Geometry: final body of the model. Coordinates: model frame, mm. Coordinates: 2 decimals unless noted, no trailing zeros. Write each loop counter-clockwise with the first axis right and the second up, starting at its lowest first coordinate (ties: lowest second). Pieces come first, ordered by that corner, then holes. Notation, with made-up numbers: (60, -15.5) - (87, -15.5) arc R30 cw to (87, 7.5) - close; hole circle Ø6 at (62, 1). An arc over 180 degrees is marked (long way). Answer as a JSON object with one key per item and string values. Group by question number.
Item 1: Section C-C on z = 40. State how many separate pieces and enclosed holes the cut face has, and give its area (3 significant figures).
Item 2: Section B-B on x = -12.75. Return loops of the section in (y, z).
Item 3: Line query: line 1 along Y through (x, z) = (-44, 44); line 2 along X through (y, z) = (-11, 47.5); line 3 along X through (y, z) = (-14.5, 12). Output: solid intervals per line, ascending. Write a range as from..to.
Item 4: Mould query, pull axis X, two halves, no side actions, for faces 1 (the cylindrical face through (-55.859, 19.961, 1.203)), 2 (the cylindrical face through (-1.203, -20.859, 36.448)), 3 (the cylindrical face through (-10.766, -14.521, 33.524)). Classes: pulls with the +X half, pulls with the -X half, needs draft (parallel to the pull), parting line crosses it, or undercut.
Item 5: Section A-A on y = 32. Return loops of the section in (x, z).
```python
from build123d import *

# Parameters (mm, degrees)
F0_R     = 2.5
F1_DEPTH = 68
F2_R     = 4


with BuildPart() as f1:
    # F0 (on Top) → F1 (new body)
    with BuildSketch(Plane.XY):
        with BuildLine():
            Line((-44.25, -10.5), (-44.25, 0))
            Line((-44.25, 0), (-57, 0))
            Line((-57, 0), (-57, -22))
            Line((-57, -22), (0, -22))
            Line((0, -22), (0, 0))
            Line((0, 0), (-28.5, 0))
            Line((-28.5, 0), (-28.5, -13))
            Line((-28.5, -13), (-41.75, -13))
            ThreePointArc((-41.75, -13), (-46.017766953, -14.767766953), (-44.25, -10.5))
        make_face()
        with BuildLine():
            ThreePointArc((-10.25, -13), (-12.75, -15.5), (-15.25, -13))
            ThreePointArc((-15.25, -13), (-12.75, -10.5), (-10.25, -13))
        make_face(mode=Mode.SUBTRACT)
        with BuildLine():
            Line((-44.25, 6.5), (-44.25, 0))
            Line((-44.25, 0), (-28.5, 0))
            Line((-28.5, 0), (0, 0))
            Line((0, 0), (0, 63))
            Line((0, 63), (-57, 63))
            Line((-57, 63), (-57, 9))
            Line((-57, 9), (-46.75, 9))
            ThreePointArc((-46.75, 9), (-44.25, 11.5), (-41.75, 9))
            ThreePointArc((-41.75, 9), (-42.482233047, 7.232233047), (-44.25, 6.5))
        make_face()
        with Locations((-12.75, 9.2245186158)):
            Circle(F0_R, mode=Mode.SUBTRACT)
        with Locations((-44.25, 32)):
            Circle(F0_R, mode=Mode.SUBTRACT)
        with BuildLine():
            ThreePointArc((-46.75, 54.2245186158), (-44.25, 56.7245186158), (-41.75, 54.2245186158))
            ThreePointArc((-41.75, 54.2245186158), (-44.25, 51.7245186158), (-46.75, 54.2245186158))
        make_face(mode=Mode.SUBTRACT)
        with Locations((-12.75, 32)):
            Circle(F0_R, mode=Mode.SUBTRACT)
        with BuildLine():
            ThreePointArc((-15.25, 54.2245186158), (-12.75, 56.7245186158), (-10.25, 54.2245186158))
            ThreePointArc((-10.25, 54.2245186158), (-12.75, 51.7245186158), (-15.25, 54.2245186158))
        make_face(mode=Mode.SUBTRACT)
        with BuildLine():
            Line((-57, 0), (-44.25, 0))
            Line((-44.25, 0), (-44.25, 6.5))
            ThreePointArc((-44.25, 6.5), (-46.017766953, 7.232233047), (-46.75, 9))
            Line((-46.75, 9), (-57, 9))
            Line((-57, 9), (-57, 0))
        make_face()
        with BuildLine():
            Line((-28.5, 0), (-44.25, 0))
            Line((-44.25, 0), (-44.25, -10.5))
            ThreePointArc((-44.25, -10.5), (-42.482233047, -11.232233047), (-41.75, -13))
            Line((-41.75, -13), (-28.5, -13))
            Line((-28.5, -13), (-28.5, 0))
        make_face()
    extrude(amount=F1_DEPTH)

    # F2
    f2_edges = [f1.edges().sort_by_distance(p)[0] for p in [
        (-28.5, 63, 0),
        (0, 20.5, 0),
        (-57, 20.5, 0),
        (-57, 63, 34),
        (0, 63, 34),
        (-28.5, -22, 0),
        (-57, -22, 34),
        (0, -22, 34),
    ]]
    fillet(f2_edges, radius=F2_R)


solid = f1.part
```
Checks:
{
 "1": {"separate pieces": "1", "enclosed holes": "8", "area": "4,670 mm^2"},
 "2": {"outline": "(-22, 4) arc R4 ccw to (-18, 0) - (-15.5, 0) - (-15.5, 68) - (-22, 68) - close; (-10.5, 0) - (6.72, 0) - (6.72, 68) - (-10.5, 68) - close; (11.72, 0) - (29.5, 0) - (29.5, 68) - (11.72, 68) - close; (34.5, 0) - (51.72, 0) - (51.72, 68) - (34.5, 68) - close; (56.72, 0) - (59, 0) arc R4 ccw to (63, 4) - (63, 68) - (56.72, 68) - close"},
 "3": {"line 1": "-22..-15.49, -10.51..6.51, 11.49..29.51, 34.49..51.74, 56.71..63", "line 2": "-57..-45.75, -42.75..-14.25, -11.25..0", "line 3": "-57..-46.25, -42.25..-14.75, -10.75..0"},
 "4": {"face 1": "pulls with the -X half", "face 2": "pulls with the +X half", "face 3": "undercut"},
 "5": {"outline": "(-57, 4) arc R4 ccw to (-53, 0) - (-46.75, 0) - (-46.75, 68) - (-57, 68) - close; (-41.75, 0) - (-15.25, 0) - (-15.25, 68) - (-41.75, 68) - close; (-10.25, 0) - (-4, 0) arc R4 ccw to (0, 4) - (0, 68) - (-10.25, 68) - close"}
}
